from build123d import *

# Parameters (mm, degrees)
SKETCH1_R           = 1.75
SKETCH1_R_2         = 1.6
SKETCH1_R_3         = 1.1
SKETCH1_R_4         = 2.1
SKETCH1_W           = 41
SKETCH1_H           = 21
SKETCH1_W_2         = 10
SKETCH1_H_2         = 3
SKETCH1_H_3         = 25
SKETCH1_W_3         = 15
SKETCH1_W_4         = 20
SKETCH1_H_4         = 10
SKETCH1_W_5         = 5
BOSS_EXTRUDE1_DEPTH = 3
FILLET1_R           = 5


with BuildPart() as part:
    # Sketch1 → Boss-Extrude1 (new body)
    with BuildSketch(Plane(origin=(0, 0, 0), x_dir=(1, 0, 0), z_dir=(0, 1, 0))):
        with BuildLine():
            Line((40, 87.5), (40, 57.5))
            Line((40, 57.5), (120, 57.5))
            Line((120, 57.5), (120, 87.5))
            Line((120, 87.5), (136.956007081, 87.5))
            ThreePointArc((136.956007081, 87.5), (150, 0), (136.956007081, -87.5))
            Line((136.956007081, -87.5), (120, -87.5))
            Line((120, -87.5), (120, -57.5))
            Line((120, -57.5), (40, -57.5))
            Line((40, -57.5), (40, -87.5))
            Line((40, -87.5), (-19.054445662, -87.5))
            Line((-19.054445662, -87.5), (-19.054445662, -77.5))
            Line((-19.054445662, -77.5), (-9.054445662, -67.5))
            Line((-9.054445662, -67.5), (-9.054445662, -57.465130862))
            Line((-9.054445662, -57.465130862), (-29.037011093, -37.482565431))
            Line((-29.037011093, -37.482565431), (-56.537011093, -37.482565431))
            Line((-56.537011093, -37.482565431), (-56.537011093, -50))
            Line((-56.537011093, -50), (-66.537011093, -50))
            Line((-66.537011093, -50), (-66.537011093, -37.482565431))
            Line((-66.537011093, -37.482565431), (-94.037011093, -37.482565431))
            Line((-94.037011093, -37.482565431), (-114.054445662, -57.5))
            Line((-114.054445662, -57.5), (-114.054445662, -67.5))
            Line((-114.054445662, -67.5), (-104.054445662, -77.5))
            Line((-104.054445662, -77.5), (-104.054445662, -87.5))
            Line((-104.054445662, -87.5), (-126.554445662, -87.5))
            ThreePointArc((-126.554445662, -87.5), (-150, 0), (-126.554445662, 87.5))
            Line((-126.554445662, 87.5), (-104.054445662, 87.5))
            Line((-104.054445662, 87.5), (-104.054445662, 77.5))
            Line((-104.054445662, 77.5), (-114.054445662, 67.5))
            Line((-114.054445662, 67.5), (-114.054445662, 57.5))
            Line((-114.054445662, 57.5), (-94.037011093, 37.482565431))
            Line((-94.037011093, 37.482565431), (-66.537011093, 37.482565431))
            Line((-66.537011093, 37.482565431), (-66.537011093, 50))
            Line((-66.537011093, 50), (-56.537011093, 50))
            Line((-56.537011093, 50), (-56.537011093, 37.482565431))
            Line((-56.537011093, 37.482565431), (-29.037011093, 37.482565431))
            Line((-29.037011093, 37.482565431), (-9.054445662, 57.465130862))
            Line((-9.054445662, 57.465130862), (-9.054445662, 67.5))
            Line((-9.054445662, 67.5), (-19.054445662, 77.5))
            Line((-19.054445662, 77.5), (-19.054445662, 87.5))
            Line((-19.054445662, 87.5), (40, 87.5))
        make_face()
        with Locations(Location((-61.537011093, 45, 0), (0, 0, 270))):
            Circle(SKETCH1_R, mode=Mode.SUBTRACT)
        with Locations(Location((-61.537011093, -45, 0), (0, 0, 90))):
            Circle(SKETCH1_R, mode=Mode.SUBTRACT)
        with Locations(Location((-100, 32.5, 0), (0, 0, 270))):
            Circle(SKETCH1_R_2, mode=Mode.SUBTRACT)
        with Locations(Location((100, 32.5, 0), (0, 0, 90))):
            Circle(SKETCH1_R_2, mode=Mode.SUBTRACT)
        with Locations(Location((100, -32.5, 0), (0, 0, 270))):
            Circle(SKETCH1_R_2, mode=Mode.SUBTRACT)
        with Locations(Location((-100, -32.5, 0), (0, 0, 90))):
            Circle(SKETCH1_R_2, mode=Mode.SUBTRACT)
        with Locations(Location((-120, -40, 0), (0, 0, 270))):
            Circle(SKETCH1_R_2, mode=Mode.SUBTRACT)
        with Locations(Location((0, -40, 0), (0, 0, 270))):
            Circle(SKETCH1_R_2, mode=Mode.SUBTRACT)
        with Locations(Location((120, -40, 0), (0, 0, 270))):
            Circle(SKETCH1_R_2, mode=Mode.SUBTRACT)
        with Locations(Location((120, 40, 0), (0, 0, 90))):
            Circle(SKETCH1_R_2, mode=Mode.SUBTRACT)
        with Locations(Location((0, 40, 0), (0, 0, 90))):
            Circle(SKETCH1_R_2, mode=Mode.SUBTRACT)
        with Locations(Location((-120, 40, 0), (0, 0, 90))):
            Circle(SKETCH1_R_2, mode=Mode.SUBTRACT)
        with Locations(Location((-137.5, 35.4, 0), (0, 0, 270))):
            Circle(SKETCH1_R_3, mode=Mode.SUBTRACT)
        with Locations(Location((-93.847011093, -4.925, 0), (0, 0, 270))):
            Circle(SKETCH1_R_4, mode=Mode.SUBTRACT)
        with Locations(Location((-93.847011093, 4.925, 0), (0, 0, 90))):
            Circle(SKETCH1_R_4, mode=Mode.SUBTRACT)
        with Locations(Location((-43.327011093, -4.925, 0), (0, 0, 90))):
            Circle(SKETCH1_R_4, mode=Mode.SUBTRACT)
        with Locations(Location((-43.327011093, 4.925, 0), (0, 0, 270))):
            Circle(SKETCH1_R_4, mode=Mode.SUBTRACT)
        with Locations(Location((-137.5, 44.6, 0), (0, 0, 270))):
            Circle(SKETCH1_R_3, mode=Mode.SUBTRACT)
        with Locations(Location((-137.5, -35.4, 0), (0, 0, 90))):
            Circle(SKETCH1_R_3, mode=Mode.SUBTRACT)
        with Locations(Location((-137.5, -44.6, 0), (0, 0, 90))):
            Circle(SKETCH1_R_3, mode=Mode.SUBTRACT)
        with Locations(Location((137.5, 35.4, 0), (0, 0, 90))):
            Circle(SKETCH1_R_3, mode=Mode.SUBTRACT)
        with Locations(Location((137.5, 44.6, 0), (0, 0, 90))):
            Circle(SKETCH1_R_3, mode=Mode.SUBTRACT)
        with Locations(Location((137.5, -35.4, 0), (0, 0, 270))):
            Circle(SKETCH1_R_3, mode=Mode.SUBTRACT)
        with Locations(Location((137.5, -44.6, 0), (0, 0, 270))):
            Circle(SKETCH1_R_3, mode=Mode.SUBTRACT)
        with Locations((-68.587011093, 0)):
            Rectangle(SKETCH1_W, SKETCH1_H, mode=Mode.SUBTRACT)
        with Locations((59.4, 36.4)):
            Rectangle(SKETCH1_W_2, SKETCH1_H_2, mode=Mode.SUBTRACT)
        with Locations((59.4, -36.4)):
            Rectangle(SKETCH1_W_2, SKETCH1_H_2, mode=Mode.SUBTRACT)
        with Locations((132.5, 0)):
            Rectangle(SKETCH1_W_2, SKETCH1_H_3, mode=Mode.SUBTRACT)
        with Locations((25, 25)):
            Rectangle(SKETCH1_W_3, SKETCH1_H_2, mode=Mode.SUBTRACT)
        with Locations((25, -25)):
            Rectangle(SKETCH1_W_3, SKETCH1_H_2, mode=Mode.SUBTRACT)
        with Locations((14, 62.5)):
            Rectangle(SKETCH1_W_4, SKETCH1_H_4, mode=Mode.SUBTRACT)
        with Locations((14, -62.5)):
            Rectangle(SKETCH1_W_4, SKETCH1_H_4, mode=Mode.SUBTRACT)
        with Locations((-125, 0)):
            Rectangle(SKETCH1_W_5, SKETCH1_H_4, mode=Mode.SUBTRACT)
    extrude(amount=BOSS_EXTRUDE1_DEPTH)

    # Fillet1
    fillet1_edges = [part.edges().sort_by_distance(p)[0] for p in [
        (120, 1.5, 57.5),
        (120, 1.5, -57.5),
        (40, 1.5, -57.5),
        (40, 1.5, -87.5),
        (-19.054445662, 1.5, -87.5),
        (40, 1.5, 57.5),
        (-56.537011093, 1.5, 37.482565431),
        (-56.537011093, 1.5, 50),
        (-66.537011093, 1.5, 50),
        (-66.537011093, 1.5, 37.482565431),
        (-56.537011093, 1.5, -37.482565431),
        (-56.537011093, 1.5, -50),
        (-66.537011093, 1.5, -50),
        (-66.537011093, 1.5, -37.482565431),
        (-94.037011093, 1.5, -37.482565431),
        (-126.554445662, 1.5, -87.5),
        (-126.554445662, 1.5, 87.5),
        (40, 1.5, 87.5),
        (-19.054445662, 1.5, 87.5),
        (-19.054445662, 1.5, 77.5),
        (-9.054445662, 1.5, 67.5),
        (-9.054445662, 1.5, 57.465130862),
        (-29.037011093, 1.5, 37.482565431),
        (-94.037011093, 1.5, 37.482565431),
        (-114.054445662, 1.5, 67.5),
        (-114.054445662, 1.5, 57.5),
        (-104.054445662, 1.5, 77.5),
        (-104.054445662, 1.5, 87.5),
        (-19.054445662, 1.5, -77.5),
        (-9.054445662, 1.5, -67.5),
        (-9.054445662, 1.5, -57.465130862),
        (-29.037011093, 1.5, -37.482565431),
        (-114.054445662, 1.5, -57.5),
        (-114.054445662, 1.5, -67.5),
        (-104.054445662, 1.5, -77.5),
        (-104.054445662, 1.5, -87.5),
        (120, 1.5, -87.5),
        (136.956007081, 1.5, -87.5),
        (136.956007081, 1.5, 87.5),
        (120, 1.5, 87.5),
    ]]
    fillet(fillet1_edges, radius=FILLET1_R - 0.0001)  # a hair under: the kernel refuses the full size


solid = part.part
Design review of the part built by this model. Coordinates are the model's own, in mm. A direction names the side the tool comes from. Round coordinates to 2 decimals unless told otherwise and drop trailing zeros. Write each loop counter-clockwise with the first axis right and the second up, starting at its lowest first coordinate (ties: lowest second). Pieces come first, ordered by that corner, then holes. Notation, with made-up numbers: (24, 1.5) -> (41, 1.5) arc R33 ccw to (41, 33.5) -> close; hole circle Ø8 at (44.5, 83). An arc over 180 degrees is marked (long way). One line per question, with ' | ' between items.
(1) Take a section at C-C, the plane y = 1.85. State how many separate pieces and enclosed holes the cut face has, and give its area (3 significant figures).
Result sheet:
separate pieces: 1 | enclosed holes: 33 | area: 34,800 mm2
(2) Wall thickness on line 1 (Z direction, x = 57, y = 2.1); line 2 (Z direction, x = 15, y = 1.3); line 3 (X direction, y = 0.55, z = -58): over which ranges is each line inside the solid? List them lowest first. Write a range as [from, to].
Result sheet:
line 1: [-57.5, -37.9], [-34.9, 34.9], [37.9, 57.5] | line 2: [-87.5, -67.5], [-57.5, 57.5], [67.5, 87.5] | line 3: [-140.11, -113.8], [-9.3, 4], [24, 42.82], [117.18, 144.34]
(3) Draft analysis for pull direction X (two halves, no side actions). For faces 1 (the flat face through (2, 3, -1)), 2 (the flat face through (-109.104, 1.479, 72.451)), 3 (the flat face through (-18.93, 1.48, 47.59)), 4 (the cylindrical face through (-149.996, 1.479, 1.241)), state which applies: released by +X, released by -X, zero draft, split by the parting line, or undercut.
Result sheet:
face 1: zero draft | face 2: undercut | face 3: undercut | face 4: released by -X
(4) Insertion check: P1, Ø0.9, axis at x = -79.5, y = 2, coming from the +Z side; P2, Ø0.9, axis at y = 1, z = 24.5, coming from the +X side; P3, Ø0.9, axis at y = 1.5, z = -61.5, coming from the +X side; P4, Ø3, axis at x = 100, z = 32.5, coming from the +Y side. Each pin has a flat end and moves straight along its axis. Give the tip position at first contact, or say it passes through.
Result sheet:
P1: z = 37.48 | P2: x = 149.03 | P3: x = 143.72 | P4: through
(5) Take a section at A-A, the plane x = 14.5. State the section outline as (y, z) points.
Result sheet:
outline: (0, -87.5) -> (3, -87.5) -> (3, -67.5) -> (0, -67.5) -> close; (0, -57.5) -> (3, -57.5) -> (3, 57.5) -> (0, 57.5) -> close; (0, 67.5) -> (3, 67.5) -> (3, 87.5) -> (0, 87.5) -> close
(6) Machinability: for faces 5 (the flat face through (-109.005, 1.479, -72.549)), 6 (the flat face through (2, 0, -1)), which of the approach directions +Z, -Z, +X, -X, +Y, -Y give a long, thin tool a straight path to every point of the face, cutting with its end or side? Answer none if there is none.
Result sheet:
face 5: +Y, -Y | face 6: +Z, -Z, +X, -X, -Y
(7) Take a section at B-B, the plane x = 87. State the section outline as (y, z) points.
Result sheet:
outline: (0, -57.5) -> (3, -57.5) -> (3, 57.5) -> (0, 57.5) -> close
